Build history of the part. All positions in model axes, mm. Face numbers are marked on the shaded views. A direction names the side the tool comes from. Give positions to 0.01 mm unless a question says otherwise; leave off trailing zeros. Write each loop counter-clockwise with the first axis right and the second up, starting at its lowest first coordinate (ties: lowest second). Pieces come first, ordered by that corner, then holes. Notation, with made-up numbers: (28.5, 50.5) -> (50.5, 50.5) arc R28 ccw to (50.5, 88.5) -> close; hole circle Ø10 at (-40, 37). An arc over 180 degrees is marked (long way). Write item = value, one per line. Start each with the question number.
Q1. Drop flat-ended pins along their axis: P1, Ø5, axis at y = -28, z = 22, coming from the +X side; P2, Ø4, axis at x = -9.5, y = 11, coming from the +Z side; P3, Ø2, axis at x = -2.5, z = 29, coming from the +Y side. Give the stop position or say it passes through.
Q2. Tool access for the marked faces 1, 2 and 3: list every direction of +Z, -Z, +X, -X, +Y, -Y with a clear straight run to the whole face (end or side of a thin tool).
Q3. Saw through at D-D, the plane z = -35. List the corners of the cut face in (x, y).
Q4. Saw through at B-B, the plane z = 28. List the corners of the cut face in (x, y).
Q5. Wall check: line 1 (X direction, y = 14, z = -8.5); line 2 (X direction, y = -21.5, z = 24); line 3 (Y direction, x = 14, z = -26). Give the ranges that are in metal, low to high.
Q6. Saw through at C-C, the plane x = 3.5. List the corners of the cut face in (y, z).
Q7. Saw through at A-A, the plane y = -4. List the corners of the cut face in (x, z), then the cut area to 3 significant figures.
Q8. Mould opens along Z. For the marked faces 4, 5 and 6 say: pulls with the +Z half, pulls with the -Z half, needs draft (parallel to the pull), parting line crosses it, or undercut.
from build123d import *

# Parameters (mm, degrees)
REVOLVE2_ANGLE = 270


with BuildPart() as part:
    # Sketch1 → Revolve2 (revolve)
    with BuildSketch(Plane.XY):
        Polygon((-10, 0), (10, 0), (10, 20), (5, 20), (5, 45), (25, 45), (25, 50), (-25, 50), (-25, 45), (-5, 45), (-5, 20), (-10, 20), align=None)
    revolve(axis=Axis((-10, 0, 0), (-1, 0, 0)), revolution_arc=REVOLVE2_ANGLE)


solid = part.part
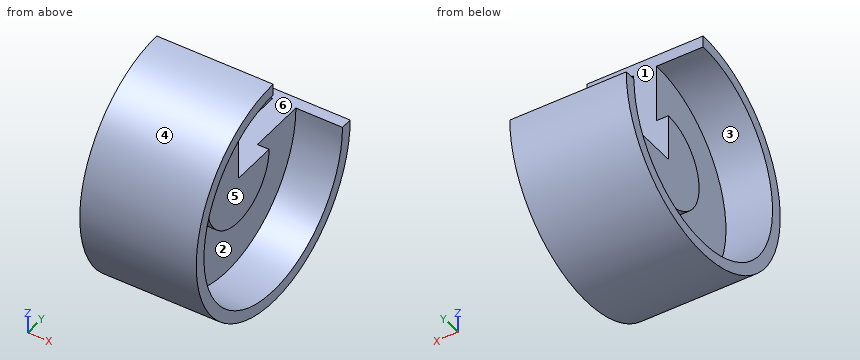
Report:
q1.P1 = 5
q1.P2 = 0
q1.P3 = 0
q2.face_1 = +Z, +X, -X, +Y
q2.face_2 = +X
q2.face_3 = -X
q3.outline = (-25, -35.71) -> (25, -35.71) -> (25, -28.28) -> (5, -28.28) -> (5, 28.28) -> (25, 28.28) -> (25, 35.71) -> (-25, 35.71) -> (-25, 28.28) -> (-5, 28.28) -> (-5, -28.28) -> (-25, -28.28) -> close
q4.outline = (-25, -41.42) -> (25, -41.42) -> (25, -35.23) -> (5, -35.23) -> (5, 0) -> (-5, 0) -> (-5, -35.23) -> (-25, -35.23) -> close
q5.line_1 = -10 to 10
q5.line_2 = -5 to 5
q5.line_3 = -42.71 to -36.73, 36.73 to 42.71
q6.outline = (0, 0) -> (0, 50) arc R50 ccw (long way) to (50, 0) -> close
q7.outline = (-25, -49.84) -> (25, -49.84) -> (25, -44.82) -> (5, -44.82) -> (5, -19.6) -> (10, -19.6) -> (10, 19.6) -> (5, 19.6) -> (5, 44.82) -> (25, 44.82) -> (25, 49.84) -> (-25, 49.84) -> (-25, 44.82) -> (-5, 44.82) -> (-5, 19.6) -> (-10, 19.6) -> (-10, -19.6) -> (-5, -19.6) -> (-5, -44.82) -> (-25, -44.82) -> close
q7.area = 1,790 mm2
q8.face_4 = parting line crosses it
q8.face_5 = undercut
q8.face_6 = pulls with the +Z half
